Autodesk Fusion 360 part; units mm, degrees
sketch "Skizze1" plane through (0, 0, 0) normal (0, 0, 1) x (1, 0, 0)
  circle A0 centre (0, 0) radius 80
extrude "Extrusion1" add sketch "Skizze1" along normal blind 10 makes body 1
fillet "Abrundung1" radius 2 1 edges at (-74.5862, -28.9292, 10) on bodies 1
sketch "Skizze2" plane through (0, 0, 0) normal (0, 1, 0) x (1, 0, 0)
  line L0 (45, 0) -> (-5, -86.6025) construction
ref_plane "Arbeitsebene1" through (-5, 0, 86.6025) normal (-0.5, 0, 0.866) x (0, -1, 0)
sketch "Skizze3" plane through (-5, 0, 86.6025) normal (-0.5, 0, 0.866) x (0, -1, 0)
  circle A0 centre (0, 0) radius 23
  circle A1 centre (0, 0) radius 20
extrude "Extrusion5" add sketch "Skizze3" against normal blind 110 separate body contours A0 | A1 makes body 2
combine "Kombinieren1" operation add target body 1 tool bodies 2
extrude "Extrusion6" cut sketch "Skizze3" against normal blind 50 bodies 1
fillet "Abrundung2" radius 4 3 edges at (65.7846, 0, 10) (-74.5862, -28.9292, 8) (-72.7215, 28.206, 10) on bodies 1
sketch "Skizze4" plane through (-5, 0, 86.6025) normal (-0.5, 0, 0.866) x (0, -1, 0)
  circle A0 centre (0, 0) radius 15.75
extrude "Extrusion7" cut sketch "Skizze4" against normal blind 110 bodies 1
sketch "Skizze5" plane through (0, 0, 0) normal (0, 0, 1) x (1, 0, 0)
  circle A0 centre (0, 0) radius 160
extrude "Extrusion8" cut sketch "Skizze5" against normal blind 110 bodies 1
ref_plane "Arbeitsebene2" through (70, 0, 0) normal (1, 0, 0) x (0, 1, 0)
sketch "Skizze6" plane through (70, 0, 0) normal (1, 0, 0) x (0, 0, -1)
  circle A0 centre (-4.5, 0) radius 3
extrude "Extrusion9" cut sketch "Skizze6" along normal mid plane 32 bodies 1
chamfer "Fase1" distance 0.3 angle 45 2 edges at (60.3709, 2.9933, 4.3029) (79.9437, -3, 4.5) on bodies 1
equation "base_plate_diameter = 160 mm"
equation "base_plate_height = 10 mm"
equation "base_plate_rounding = 2 mm"
equation "leg_outer_diameter = 46 mm"
equation "ring_inner_diameter = 40 mm"
equation "ring_extrude_depth = 50 mm"
equation "hole_inner_diameter = 31.5 mm"
equation "leg_length = 100 mm"
equation "leg_angle = 120 deg"
equation "leg_offset = 45 mm"
equation "leg_plate_rounding = 4 mm"
equation "cable_hole_offset = 70 mm"
equation "cable_hole_diameter = 6 mm"
equation "cable_hole_height = 4.5 mm"
equation "cable_hole_chamfer = 0.3 mm"
equation "d16 = base_plate_height"
equation "d19 = base_plate_rounding"
equation "d32 = leg_plate_rounding"
equation "d41 = cable_hole_chamfer"
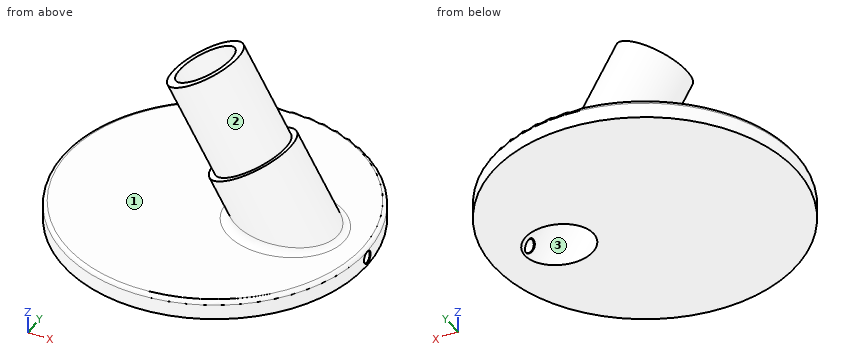
Input: part model. Units: mm. Frame: model coordinates. Face numbers are marked on the shaded views. Give positions to 0.01 mm unless a question says otherwise; leave off trailing zeros. Answer as a JSON object with one key per item and string values.
1. Ray query, line 1 (Z direction, x = 72, y = 0); line 2 (Z direction, x = 38.5, y = 60); line 3 (Y direction, x = 64.5, z = 4.5). Return the intervals inside material, ascending. Write a range as [from, to].
Result sheet:
{"line 1": "[0, 1.5], [7.5, 10]", "line 2": "[0, 10]", "line 3": "[-47.33, -3], [3, 47.33]"}
2. First-contact query: P1, Ø1, axis at x = 4, z = 48.5, coming from the +Y side; P2, Ø1.5, axis at x = -48.5, y = -8, coming from the +Z side; P3, Ø1.5, axis at y = -18, z = 77, coming from the +X side. Flat tips, straight axial feed; report the tip coordinate or a pass-through.
Result sheet:
{"P1": "y = 16.86", "P2": "z = 10", "P3": "x = 12.29"}
3. Pull-direction query (Y, two-part tool) for the marked faces 1, 2 and 3; classes: +Y half, -Y half, draft (parallel to the pull), parting line (faces both ways), or undercut.
Result sheet:
{"face 1": "draft", "face 2": "parting line", "face 3": "undercut"}
